Here's how the part is built. I have some questions about the finished solid (model axes, mm). Face numbers are marked on the shaded views. A direction names the side the tool comes from. Coordinates: 2 decimals unless noted, no trailing zeros. Order: outer loops, then holes, each group sorted by start corner. A loop starts at its lowest first (then second) coordinate and runs counter-clockwise, first axis right, second up. Notation, with made-up numbers: (-2, 29.5) - (49, 29.5) arc R28 cw to (49, 57.5) - close; hole circle Ø10 at (-12.5, 8). An arc over 180 degrees is marked (long way). Answer in a Markdown table with one row per item. Add a question column.
Item 1: Will these pins go through, and if not, where does the flat tip stop? pin 1 Ø1 at (y, z) = (3, 1.5) entering from -X; pin 2 Ø1.5 at (x, z) = (1.5, 0) entering from -Y; pin 3 Ø1 at (y, z) = (0.5, 5) entering from +X.
Item 2: If I drill on line 1 along X through (y, z) = (-0.25, -1); line 2 along Y through (x, z) = (-1.25, 2.5); line 3 along Y through (x, z) = (-0.5, 11) (3 decimals), over which ranges is the centre line in solid material (lowest first)? Write a range as from..to.
Item 3: I want a section at D-D (z = -0.75). Please give me the cut outline in (x, y), plus the area to 3 significant figures.
Item 4: I want a section at B-B (z = 12). Please give me the cut outline in (x, y).
Item 5: I want a section at C-C (x = 0). Please give me the cut outline in (y, z), plus the area to 3 significant figures.
Item 6: On a 3-axis mill with a long thin cutter (end or side, diameter ignored), from which of +Z, -Z, +X, -X, +Y, -Y can I reach the whole of each face in a straight line? I mean the marked faces 1, 2 and 3. Say none if no direction works.
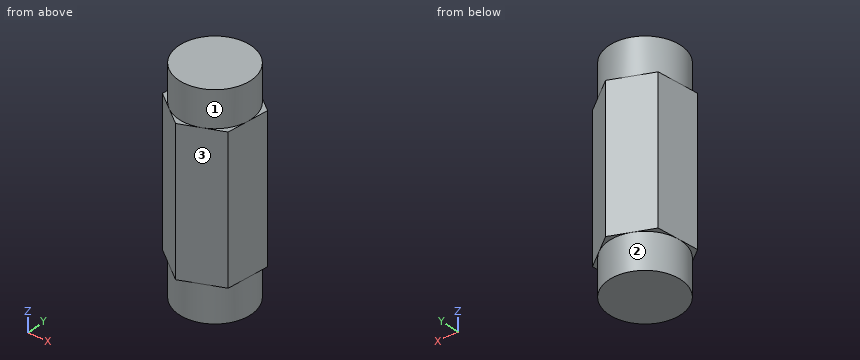
```python
from build123d import *

# Parameters (mm, degrees)
EXTRUDE_2_DEPTH = 20
SKETCH_2_R      = 5
EXTRUDE_3_DEPTH = 5
EXTRUDE_START   = 5
SKETCH_3_R      = 5
EXTRUDE_4_DEPTH = 5


with BuildPart() as part:
    # 草图1 → 凸台-拉伸2 (new body)
    with BuildSketch(Plane.XY):
        Polygon((5.3293871, 2.220577958), (0.741616627, 5.725673595), (-4.587770473, 3.505095636), (-5.3293871, -2.220577958), (-0.741616627, -5.725673595), (4.587770473, -3.505095636), align=None)
    extrude(amount=EXTRUDE_2_DEPTH)

    # 草图2 → 凸台-拉伸3 (add)
    with BuildSketch(Plane(origin=(0, 0, 0), x_dir=(-1, 0, 0), z_dir=(0, 0, -1))):
        with Locations(Location((0, 0, 0), (0, 0, 187.380135052))):
            Circle(SKETCH_2_R)
    extrude(amount=EXTRUDE_3_DEPTH)

    # 草图3 → 凸台-拉伸4 (add)
    with BuildSketch(Plane.XY.offset(20).offset(EXTRUDE_START)):
        with Locations(Location((0, 0, 0), (0, 0, 352.619864948))):
            Circle(SKETCH_3_R)
    extrude(amount=-EXTRUDE_4_DEPTH)


solid = part.part
```
Values follow:
| question | item | result |
|---|---|---|
| 1 | pin 1 | stops at x = -4.72 |
| 1 | pin 2 | stops at y = -5.1 |
| 1 | pin 3 | stops at x = 5.17 |
| 2 | line 1 | x = -4.99..4.99 |
| 2 | line 2 | y = -5.34..4.9 |
| 2 | line 3 | y = -5.625..5.208 |
| 3 | outline | circle Ø10 at (0, 0) |
| 3 | area | 78.5 mm^2 |
| 4 | outline | (-5.33, -2.22) - (-0.74, -5.73) - (4.59, -3.51) - (5.33, 2.22) - (0.74, 5.73) - (-4.59, 3.51) - close |
| 5 | outline | (-5.42, 0) - (-5, 0) - (-5, -5) - (5, -5) - (5, 0) - (5.42, 0) - (5.42, 20) - (5, 20) - (5, 25) - (-5, 25) - (-5, 20) - (-5.42, 20) - close |
| 5 | area | 317 mm^2 |
| 6 | face 1 | +Z |
| 6 | face 2 | -Z |
| 6 | face 3 | +Z, -Z, +X, -Y |
